```python
from build123d import *

# Parameters (mm, degrees)
BOSS_EXTRUDE1_DEPTH             = 12.2
SKETCH2_W                       = 2
SKETCH2_H                       = 26
CUT_EXTRUDE1_DEPTH              = 43
SKETCH3_W                       = 26
SKETCH3_H                       = 2
CUT_EXTRUDE2_DEPTH              = 43
SKETCH4_R                       = 16.5
CUT_EXTRUDE3_DEPTH              = 0.6
SKETCH5_R                       = 11
BOSS_EXTRUDE2_DEPTH             = 2.6
SKETCH6_R                       = 3.25
CUT_EXTRUDE4_DEPTH              = 2
SKETCH7_R                       = 2.5
CUT_EXTRUDE5_DEPTH              = 13.2
FILLET1_R                       = 0.5
FILLET3_R                       = 0.5
FILLET4_R                       = 2
M3X0_5_TAPPED_HOLE1_D           = 3
M3X0_5_TAPPED_HOLE1_DEPTH       = 10
M3X0_5_TAPPED_HOLE1_CSINK_D     = 3.5
M3X0_5_TAPPED_HOLE1_CSINK_ANGLE = 90
M3X0_5_TAPPED_HOLE1_TIP         = 0.901290929


with BuildPart() as part:
    # Sketch1 → Boss-Extrude1 (new body)
    with BuildSketch(Plane.XY):
        Polygon((-17.183766184, 21), (-21, 17.183766184), (-21, -17.183766184), (-17.183766184, -21), (17.183766184, -21), (21, -17.183766184), (21, 17.183766184), (17.183766184, 21), align=None)
    extrude(amount=BOSS_EXTRUDE1_DEPTH)

    # Sketch2 → Cut-Extrude1 (cut, through all)
    with BuildSketch(Plane(origin=(21, 0, 0), x_dir=(0, 0, -1), z_dir=(1, 0, 0))):
        with Locations((-11.2, 0)):
            Rectangle(SKETCH2_W, SKETCH2_H)
    extrude(amount=-CUT_EXTRUDE1_DEPTH, mode=Mode.SUBTRACT)

    # Sketch3 → Cut-Extrude2 (cut, through all)
    with BuildSketch(Plane(origin=(0, 21, 0), x_dir=(1, 0, 0), z_dir=(0, 1, 0))):
        with Locations((0, -11.2)):
            Rectangle(SKETCH3_W, SKETCH3_H)
    extrude(amount=-CUT_EXTRUDE2_DEPTH, mode=Mode.SUBTRACT)

    # Sketch4 → Cut-Extrude3 (cut)
    with BuildSketch(Plane(origin=(0, 0, 0), x_dir=(-1, 0, 0), z_dir=(0, 0, -1))):
        Circle(SKETCH4_R)
    extrude(amount=-CUT_EXTRUDE3_DEPTH, mode=Mode.SUBTRACT)

    # Sketch5 → Boss-Extrude2 (add)
    with BuildSketch(Plane(origin=(0, 0, 0.6), x_dir=(-1, 0, 0), z_dir=(0, 0, -1))):
        Circle(SKETCH5_R)
    extrude(amount=BOSS_EXTRUDE2_DEPTH)

    # Sketch6 → Cut-Extrude4 (cut)
    with BuildSketch(Plane(origin=(0, 0, -2), x_dir=(-1, 0, 0), z_dir=(0, 0, -1))):
        Circle(SKETCH6_R)
    extrude(amount=-CUT_EXTRUDE4_DEPTH, mode=Mode.SUBTRACT)

    # Sketch7 → Cut-Extrude5 (cut, through all)
    with BuildSketch(Plane(origin=(0, 0, 0), x_dir=(-1, 0, 0), z_dir=(0, 0, -1))):
        Circle(SKETCH7_R)
    extrude(amount=-CUT_EXTRUDE5_DEPTH, mode=Mode.SUBTRACT)

    # Fillet1
    fillet1_edges = [part.edges().sort_by_distance(p)[0] for p in [
        (3.25, 0, -2),
    ]]
    fillet(fillet1_edges, radius=FILLET1_R)

    # Fillet3
    fillet3_edges = [part.edges().sort_by_distance(p)[0] for p in [
        (11, 0, 0.6),
    ]]
    fillet(fillet3_edges, radius=FILLET3_R)

    # Fillet4
    fillet4_edges = [part.edges().sort_by_distance(p)[0] for p in [
        (17.183766184, 21, 6.1),
        (21, 17.183766184, 6.1),
        (21, -17.183766184, 6.1),
        (17.183766184, -21, 6.1),
        (-17.183766184, -21, 6.1),
        (-21, -17.183766184, 6.1),
        (-21, 17.183766184, 6.1),
        (-17.183766184, 21, 6.1),
    ]]
    fillet(fillet4_edges, radius=FILLET4_R)

    # M3x0.5 Tapped Hole1
    with Locations(Plane(origin=(0, 0, 0), x_dir=(-1, 0, 0), z_dir=(0, 0, -1))):
        with Locations((-15.5, -15.5), (-15.5, 15.5), (15.5, 15.5), (15.5, -15.5)):
            CounterSinkHole(M3X0_5_TAPPED_HOLE1_D / 2, M3X0_5_TAPPED_HOLE1_CSINK_D / 2, depth=M3X0_5_TAPPED_HOLE1_DEPTH, counter_sink_angle=M3X0_5_TAPPED_HOLE1_CSINK_ANGLE)
            with Locations((0, 0, -(M3X0_5_TAPPED_HOLE1_DEPTH + M3X0_5_TAPPED_HOLE1_TIP / 2))):  # 118° drill point
                Cone(0, M3X0_5_TAPPED_HOLE1_D / 2, M3X0_5_TAPPED_HOLE1_TIP, mode=Mode.SUBTRACT)


solid = part.part
```
Could you check a few things on this model? Use its own coordinates, in mm. A direction names the side the tool comes from. Coordinates: 2 decimals unless noted, no trailing zeros. Order: outer loops, then holes, each group sorted by start corner. A loop starts at its lowest first (then second) coordinate and runs counter-clockwise, first axis right, second up. Notation, with made-up numbers: M 69,-12.75 L 104,-12.75 A18 ccw 104,-7.75 Z; hole C 33,28.25 d9. An arc over 180 degrees is marked long. Use one line per item in the form item = value. Start each with the question number.
1. We'd pull the mould along Y, two halves only. Please class faces 4 (the conical face through (15.38, -15.731, 10.745)), 5 (the cylindrical face through (-20.85, -17.11, 6.19)), 6 (the cylindrical face through (20.844, 17.131, 6.185)): +Y half, -Y half, draft (parallel to the pull), parting line (faces both ways), or undercut.
2. Suppose I cut it at C-C on x = 12. Write out the boundary of the cut face in (y, z), then the cut area to 3 significant figures.
3. Suppose I cut it at B-B on z = 4. Write out the boundary of the cut face in (x, y), then the cut area to 3 significant figures.
4. On a 3-axis mill with a long thin cutter (end or side, diameter ignored), from which of +Z, -Z, +X, -X, +Y, -Y can I reach the whole of each face in a straight line? I mean faces 1 (the flat face through (13, -17, 11)), 2 (the cylindrical face through (-17, -15.43, 5.19)), 3 (the flat face through (17, 13, 11)). Say none if no direction works.
5. For pin 1 (2 mm diameter, centred on x = -1.5, y = 11, fed in from +Z); pin 2 (4 mm diameter, centred on x = 0, y = 0, fed in from +Z); pin 3 (1.8 mm diameter, centred on x = 15.5, y = -15.5, fed in from -Z); pin 4 (2 mm diameter, centred on x = -18.5, z = 11, fed in from -Y), each with a flat end and sliding along its axis, tell me the tip position at first contact or that it passes through.
6. Suppose I cut it at A-A on x = 0. Write out the boundary of the cut face in (y, z), then the cut area to 3 significant figures.
7. Please list where these lines run through material, in increasing order: line 1 (Y direction, x = -15.5, z = 5.75); line 2 (Y direction, x = 0, z = -0.35).
Geometry says:
q1.face_4 = undercut
q1.face_5 = -Y half
q1.face_6 = +Y half
q2.outline = M -21,0 L -11.32,0 L -11.32,0.6 L 11.32,0.6 L 11.32,0 L 21,0 L 21,10.2 L -21,10.2 Z
q2.area = 415 mm^2
q3.outline = M -21,-16.36 A2 ccw -20.41,-17.77 L -17.77,-20.41 A2 ccw -16.36,-21 L 16.36,-21 A2 ccw 17.77,-20.41 L 20.41,-17.77 A2 ccw 21,-16.36 L 21,16.36 A2 ccw 20.41,17.77 L 17.77,20.41 A2 ccw 16.36,21 L -16.36,21 A2 ccw -17.77,20.41 L -20.41,17.77 A2 ccw -21,16.36 Z; hole C -15.5,-15.5 d3; hole C -15.5,15.5 d3; hole C 0,0 d5; hole C 15.5,-15.5 d3; hole C 15.5,15.5 d3
q3.area = 1,690 mm^2
q4.face_1 = +Z, +Y, -Y
q4.face_2 = -Z
q4.face_3 = +Z, +X, -X
q5.pin_1 = 10.2
q5.pin_2 = through
q5.pin_3 = 10.36
q5.pin_4 = -20.64
q6.outline = M -21,0 L -16.5,0 L -16.5,0.6 L -11.5,0.6 A0.5 cw -11,0.1 L -11,-2 L -3.75,-2 A0.5 ccw -3.25,-1.5 L -3.25,0 L -2.5,0 L -2.5,10.2 L -21,10.2 Z; M 2.5,0 L 3.25,0 L 3.25,-1.5 A0.5 ccw 3.75,-2 L 11,-2 L 11,0.1 A0.5 cw 11.5,0.6 L 16.5,0.6 L 16.5,0 L 21,0 L 21,10.2 L 2.5,10.2 Z
q6.area = 402 mm^2
q7.line_1 = -21 to -17, -14 to 14, 17 to 21
q7.line_2 = -11 to -3.25, 3.25 to 11
